The model under review builds one solid part; all positions refer to its coordinate system, in mm. Face numbers are marked on the shaded views. A direction names the side the tool comes from. Round coordinates to 2 decimals unless told otherwise and drop trailing zeros. Order: outer loops, then holes, each group sorted by start corner. A loop starts at its lowest first (then second) coordinate and runs counter-clockwise, first axis right, second up. Notation, with made-up numbers: (69.5, 38.5) -> (85.5, 38.5) arc R29 ccw to (85.5, 75.5) -> close; hole circle Ø9 at (22, 46.25). An arc over 180 degrees is marked (long way). Use a Markdown table: item, result. Add a question column.
```python
from build123d import *

# Parameters (mm, degrees)
F1_DEPTH = 25.4


with BuildPart() as f1:
    # F0 (on Top) → F1 (new body)
    with BuildSketch(Plane.XY):
        with BuildLine():
            Line((2.8403762262, 45.6520467997), (-73.6027508974, 45.6520467997))
            Line((-73.6027508974, 45.6520467997), (-73.6027508974, -185.4493916035))
            add(Edge.make_bspline(
                [(-9.3509247527, -182.7207505703), (-17.437708134, -190.6869860397), (-39.462107573, -194.4763575001), (-62.4702088535, -188.2325261831), (-73.6027508974, -185.4493916035)],
                knots=[0, 0, 0, 0, 0.4843647, 1, 1, 1, 1], degree=3))
            Line((-9.3509247527, -182.7207505703), (-9.3509247527, -127.6174634695))
            Line((-9.3509247527, -127.6174634695), (11.9979763404, -191.7036473751))
            add(Edge.make_bspline(
                [(90.9340977669, -192.5606280565), (78.2585442066, -189.655855298), (51.9474674394, -179.7068423852), (25.4845232477, -188.0636329791), (11.9979763404, -191.7036473751)],
                knots=[0, 0, 0, 0, 0.4967823227, 1, 1, 1, 1], degree=3))
            Line((90.9340977669, -192.5606280565), (90.9340977669, 45.6520467997))
            Line((90.9340977669, 45.6520467997), (25.5670342594, 45.6520467997))
            Line((25.5670342594, 45.6520467997), (25.5670342594, -19.4191858172))
            Line((25.5670342594, -19.4191858172), (2.8403762262, 45.6520467997))
        make_face()
        with BuildLine():
            Line((-61.6082288325, -176.0364919901), (-61.6082288325, -165.4586195946))
            add(Edge.make_bspline(
                [(-23.6730482429, -165.5816286802), (-29.6743388581, -167.1716020854), (-41.866855763, -170.422804665), (-54.9348358498, -167.1372714885), (-61.6082288325, -165.4586195946)],
                knots=[0, 0, 0, 0, 0.4892970389, 1, 1, 1, 1], degree=3))
            Line((-23.6730482429, -165.5816286802), (-23.6730482429, -176.7938733101))
            add(Edge.make_bspline(
                [(-61.6082288325, -176.0364919901), (-55.8519269533, -178.1175226352), (-44.0650777342, -182.250968639), (-30.3064212203, -179.3696731329), (-23.6730482429, -176.7938733101)],
                knots=[0, 0, 0, 0, 0.4842057013, 1, 1, 1, 1], degree=3))
        make_face(mode=Mode.SUBTRACT)
        with BuildLine():
            Line((-61.4957623184, -158.8420271873), (-61.4957623184, -147.6238518953))
            add(Edge.make_bspline(
                [(-23.566477932, -147.2548544407), (-29.712963668, -149.3360042131), (-42.0451974231, -153.5501506553), (-55.0127920336, -149.6146560989), (-61.4957623184, -147.6238518953)],
                knots=[0, 0, 0, 0, 0.494682972, 1, 1, 1, 1], degree=3))
            Line((-23.566477932, -147.2548544407), (-23.566477932, -158.9123904705))
            add(Edge.make_bspline(
                [(-61.4957623184, -158.8420271873), (-55.5822802874, -161.0065351502), (-43.5958322945, -165.2473219714), (-29.5886882908, -161.9094118541), (-23.566477932, -158.9123904705)],
                knots=[0, 0, 0, 0, 0.4898045376, 1, 1, 1, 1], degree=3))
        make_face(mode=Mode.SUBTRACT)
        with BuildLine():
            Line((22.3441086709, -176.2591153383), (19.1280748695, -166.8069213629))
            add(Edge.make_bspline(
                [(19.1280748695, -166.8069213629), (27.9156584293, -163.297533989), (45.8218010204, -157.4179008912), (66.4390050953, -162.4391177875), (76.7182558775, -165.3293818235)],
                knots=[0, 0, 0, 0, 0.4844139256, 1, 1, 1, 1], degree=3))
            Line((76.7182558775, -165.3293818235), (76.7182558775, -175.7957041264))
            add(Edge.make_bspline(
                [(22.3441086709, -176.2591153383), (30.8734351647, -173.63505248), (48.372189716, -168.6907809082), (67.1033187619, -173.3021776491), (76.7182558775, -175.7957041264)],
                knots=[0, 0, 0, 0, 0.4893730261, 1, 1, 1, 1], degree=3))
        make_face(mode=Mode.SUBTRACT)
        with BuildLine():
            add(Edge.make_bspline(
                [(17.680067569, -162.0491892099), (25.8568657938, -159.2836448096), (43.3363572549, -153.246674733), (65.3150252677, -158.0651620078), (76.8111720681, -160.4368239641)],
                knots=[0, 0, 0, 0, 0.4679630835, 1, 1, 1, 1], degree=3))
            Line((17.680067569, -162.0491892099), (13.6130254536, -150.2377683718))
            add(Edge.make_bspline(
                [(76.8111720681, -149.223998189), (65.8089509547, -146.5744464182), (44.0946442795, -141.1555049391), (23.7747255115, -147.4399738598), (13.6130254536, -150.2377683718)],
                knots=[0, 0, 0, 0, 0.5076708413, 1, 1, 1, 1], degree=3))
            Line((76.8111720681, -149.223998189), (76.8111720681, -160.4368239641))
        make_face(mode=Mode.SUBTRACT)
        with BuildLine():
            add(Edge.make_bspline(
                [(-61.3580606878, -141.6363418102), (-55.1243719971, -143.5797285758), (-42.5699592819, -147.4936358513), (-29.8592976922, -143.1950838215), (-23.4599076211, -141.0309076309)],
                knots=[0, 0, 0, 0, 0.4965336756, 1, 1, 1, 1], degree=3))
            Line((-61.3580606878, -141.6363418102), (-61.3580606878, 33.189624548))
            Line((-61.3580606878, 33.189624548), (-6.8358113058, 33.189624548))
            Line((-6.8358113058, 33.189624548), (38.6858433485, -108.5935905576))
            Line((38.6858433485, -108.5935905576), (38.6858433485, 32.2056338191))
            Line((38.6858433485, 32.2056338191), (76.8895372748, 32.2056338191))
            Line((76.8895372748, 32.2056338191), (76.8895372748, -143.5442268848))
            add(Edge.make_bspline(
                [(76.8895372748, -143.5442268848), (66.1581754684, -139.7765427828), (44.92542678, -135.6920583397), (22.2354233265, -140.7641023397), (11.9839739054, -145.3826874495)],
                knots=[0, 0, 0, 0, 0.4966206681, 1, 1, 1, 1], degree=3))
            Line((11.9839739054, -145.3826874495), (6.3145500608, -130.9114247561))
            Line((6.3145500608, -130.9114247561), (15.9579180181, -132.8547745943))
            Line((15.9579180181, -132.8547745943), (-9.0975156054, -93.8023552299))
            Line((-9.0975156054, -93.8023552299), (6.9675748236, -96.3511392474))
            Line((6.9675748236, -96.3511392474), (-13.3098065853, -59.8137304187))
            Line((-13.3098065853, -59.8137304187), (-4.043716006, -62.948577106))
            Line((-4.043716006, -62.948577106), (-20.9504030645, -27.0268172026))
            Line((-20.9504030645, -27.0268172026), (-38.7236736715, -65.0239139795))
            Line((-38.7236736715, -65.0239139795), (-29.1993748397, -61.4539980888))
            Line((-29.1993748397, -61.4539980888), (-49.4690351188, -97.7168679237))
            Line((-49.4690351188, -97.7168679237), (-33.7521508336, -95.6219658256))
            Line((-33.7521508336, -95.6219658256), (-56.8872727454, -132.2386860847))
            add(Edge.make_bspline(
                [(-56.8872727454, -132.2386860847), (-51.9440866881, -130.4241960282), (-41.8102623942, -127.6231875659), (-23.5047530606, -127.3379553592), (-23.4599076211, -127.2974461317)],
                knots=[0, 0, 0, 0, 0.4990520903, 0.9673944803, 0.9673944803, 0.9673944803, 0.9673944803], degree=3))
            Line((-23.4599076211, -127.2974461317), (-23.4599076211, -141.0309076309))
        make_face(mode=Mode.SUBTRACT)
    extrude(amount=F1_DEPTH)


solid = f1.part
```
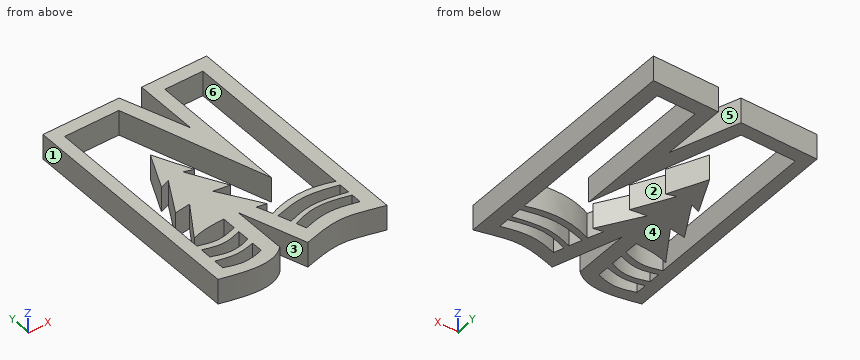
Q1. Insertion check: pin 1 (3 mm diameter, centred on x = 12.5, z = 22, fed in from -Y); pin 2 (2 mm diameter, centred on x = -55.5, z = 17, fed in from -Y); pin 3 (12.5 mm diameter, centred on x = 57, z = 10, fed in from -Y). Each pin has a flat end and moves straight along its axis. Give the tip position at first contact, or say it passes through.
Q2. Wall thickness on line 1 (X direction, y = -10.5, z = 3); line 2 (Y direction, x = 43, z = 12); line 3 (X direction, y = -110.5, z = 22.5): over which ranges is each line inside the solid? List them lowest first. Write a range as [from, to].
Q3. Add section B-B (y = -114). Write out the cut boundary in (x, z).
Q4. Mouldability with a two-part tool opening along Y and no side actions: class the marked faces 4, 5 and 6 as pulls with the +Y half, pulls with the -Y half, needs draft (parallel to the pull), parting line crosses it, or undercut.
Q5. Machinability: for the marked faces 1, 2 and 3, which of the approach directions +Z, -Z, +X, -X, +Y, -Y give a long, thin tool a straight path to every point of the face, cutting with its end or side? Answer none if there is none.
Q6. Add section C-C (x = 0.5). Write out the cut boundary in (y, z).
Q7. Add section D-D (z = 23). State how many separate pieces and enclosed holes the cut face has, then the cut area to 3 significant figures.
Q8. Add section A-A (y = 16). Write out the cut boundary in (x, z), then the cut area to 3 significant figures.
Report:
| question | item | result |
|---|---|---|
| 1 | pin 1 | stops at y = -191.7 |
| 1 | pin 2 | stops at y = -189.97 |
| 1 | pin 3 | stops at y = -185.6 |
| 2 | line 1 | x = [-73.6, -61.36], [7.19, 22.45], [25.57, 38.69], [76.89, 90.93] |
| 2 | line 2 | y = [-184.65, -171.42], [-160.33, -156.02], [-144.13, -138.03], [32.21, 45.65] |
| 2 | line 3 | x = [-73.6, -61.36], [-43.15, 1.62], [76.89, 90.93] |
| 3 | outline | (-73.6, 0) -> (-61.36, 0) -> (-61.36, 25.4) -> (-73.6, 25.4) -> close; (-45.36, 0) -> (3.86, 0) -> (3.86, 25.4) -> (-45.36, 25.4) -> close; (76.89, 0) -> (90.93, 0) -> (90.93, 25.4) -> (76.89, 25.4) -> close |
| 4 | face 4 | needs draft |
| 4 | face 5 | pulls with the +Y half |
| 4 | face 6 | undercut |
| 5 | face 1 | +Z, -Z, -X, +Y, -Y |
| 5 | face 2 | +Z, -Z |
| 5 | face 3 | +Z, -Z, -Y |
| 6 | outline | (-157.19, 0) -> (-108.76, 0) -> (-108.76, 25.4) -> (-157.19, 25.4) -> close; (-95.33, 0) -> (-84.7, 0) -> (-84.7, 25.4) -> (-95.33, 25.4) -> close; (10.34, 0) -> (45.65, 0) -> (45.65, 25.4) -> (10.34, 25.4) -> close |
| 7 | separate pieces | 1 |
| 7 | enclosed holes | 5 |
| 7 | area | 17,800 mm² |
| 8 | outline | (-73.6, 0) -> (-61.36, 0) -> (-61.36, 25.4) -> (-73.6, 25.4) -> close; (-1.32, 0) -> (13.2, 0) -> (13.2, 25.4) -> (-1.32, 25.4) -> close; (25.57, 0) -> (38.69, 0) -> (38.69, 25.4) -> (25.57, 25.4) -> close; (76.89, 0) -> (90.93, 0) -> (90.93, 25.4) -> (76.89, 25.4) -> close |
| 8 | area | 1,370 mm² |
